Part model, mm, in its own coordinate system. A direction names the side the tool comes from. Round coordinates to 2 decimals unless told otherwise and drop trailing zeros. Loops run counter-clockwise (first coordinate to the right, second up) from the corner with the lowest first, then second, coordinate; pieces in that order, holes last.
1) Drop flat-ended pins along their axis: P1, Ø5.5, axis at x = -151.9, y = 9.59, coming from the -Z side; P2, Ø3, axis at y = -30.5, z = 19.5, coming from the +X side; P3, Ø2, axis at y = -24, z = 5.5, coming from the -X side; P4, Ø5.5, axis at x = -202.89, y = 41.4, coming from the +Z side. Give the stop position or say it passes through.
2) Band-saw the part on A-A, the plane z = 22. Write the cut outline in (x, y), then the cut area to 3 significant figures.
3) Mould opens along X. For faces 3 (the flat face through (-238.316, -10.619, 13.681)), 4 (the flat face through (-30, 12, 30)) say: +X half, -X half, draft (parallel to the pull), parting line (faces both ways), or undercut.
4) 3-axis set-ups, long thin cutter, end or side, ignore diameter. For faces 1 (the flat face through (18, 12, 0)), 2 (the flat face through (-193, 1, 27.75)): which of +Z, -Z, +X, -X, +Y, -Y reach the whole face in a straight line?
5) Probe line 1 (X direction, y = -2.5, z = 12); line 2 (Y direction, x = -189, z = 11); line 3 (X direction, y = -40, z = 24). List the from-to ranges inside material, lowest first.
6) Band-saw the part on B-B, the plane x = 116. Write the cut outline in (y, z).
7) Band-saw the part on C-C, the plane x = 17. Write the cut outline in (y, z), then the cut area to 3 significant figures.
from build123d import *

# Parameters (mm, degrees)
EXTRUDE_3_DEPTH     = 30
CUT_EXTRUDE_1_DEPTH = 27.75
SKETCH_5_R          = 1.75
CUT_EXTRUDE_2_DEPTH = 250.931131666


with BuildPart() as part:
    # 草图1 → 凸台-拉伸3 (new body)
    with BuildSketch(Plane.XY):
        with BuildLine():
            ThreePointArc((188.956439237, 0), (176.309013441, 23.14413618), (150, 25))
            Line((150, 25), (150, -25))
            ThreePointArc((150, -25), (176.309013441, -23.14413618), (188.956439237, 0))
        make_face()
        with BuildLine():
            Line((150, -25), (150, 25))
            ThreePointArc((150, 25), (133.956439237, 0), (150, -25))
        make_face()
        with BuildLine():
            ThreePointArc((188.956439237, 0), (176.309013441, 23.14413618), (150, 25))
            Line((150, 25), (150, -25))
            ThreePointArc((150, -25), (176.309013441, -23.14413618), (188.956439237, 0))
        make_face()
        with BuildLine():
            Line((150, -25), (150, 25))
            ThreePointArc((150, 25), (133.956439237, 0), (150, -25))
        make_face()
        with BuildLine():
            Line((150, 25), (-150, 25))
            ThreePointArc((-150, 25), (-145.004978875, 12.940952255), (-143.301270189, 0))
            ThreePointArc((-143.301270189, 0), (-145.004978875, -12.940952255), (-150, -25))
            ThreePointArc((-150, -25), (0, -7.455532034), (150, -25))
            ThreePointArc((150, -25), (133.956439237, 0), (150, 25))
        make_face()
        with BuildLine():
            ThreePointArc((-150, 25), (0, 41.260283441), (150, 25))
            Line((150, 25), (-150, 25))
        make_face()
        with BuildLine():
            ThreePointArc((-143.301270189, 0), (-145.004978875, 12.940952255), (-150, 25))
            Line((-150, 25), (-150, -25))
            ThreePointArc((-150, -25), (-145.004978875, -12.940952255), (-143.301270189, 0))
        make_face()
        with BuildLine():
            Line((-150, -25), (-150, 25))
            ThreePointArc((-150, 25), (-243.301270189, 0), (-150, -25))
        make_face()
        with BuildLine():
            ThreePointArc((-143.301270189, 0), (-145.004978875, 12.940952255), (-150, 25))
            Line((-150, 25), (-150, -25))
            ThreePointArc((-150, -25), (-145.004978875, -12.940952255), (-143.301270189, 0))
        make_face()
        with BuildLine():
            Line((-150, -25), (-150, 25))
            ThreePointArc((-150, 25), (-243.301270189, 0), (-150, -25))
        make_face()
    extrude(amount=EXTRUDE_3_DEPTH)

    # 草图3 → 切除-拉伸1 (cut)
    with BuildSketch(Plane(origin=(0, 0, 0), x_dir=(-1, 0, 0), z_dir=(0, 0, -1))):
        with BuildLine():
            ThreePointArc((241.460241998, 2.962420354), (203.950254971, 47.06019149), (151.10937756, 23.40740687))
            Line((151.10937756, 23.40740687), (145.115292459, -2.484763599))
            ThreePointArc((145.115292459, -2.484763599), (182.186192507, -46.952290127), (235.258997062, -23.8246019))
            Line((235.258997062, -23.8246019), (238.35961953, -10.431090773))
            Line((238.35961953, -10.431090773), (241.460241998, 2.962420354))
        make_face()
    extrude(amount=-CUT_EXTRUDE_1_DEPTH, mode=Mode.SUBTRACT)

    # 草图5 → 切除-拉伸2 (cut, through all)
    with BuildSketch(Plane(origin=(0, 0, 27.75), x_dir=(-1, 0, 0), z_dir=(0, 0, -1))):
        with Locations((151.896300525, 9.585326657)):
            Circle(SKETCH_5_R)
        with Locations((170.801384844, 36.055584303)):
            Circle(SKETCH_5_R)
        with Locations((202.886596846, 41.404969664)):
            Circle(SKETCH_5_R)
        with Locations((229.356854492, 22.499885346)):
            Circle(SKETCH_5_R)
        with Locations((234.706239853, -9.585326656)):
            Circle(SKETCH_5_R)
        with Locations((215.801155535, -36.055584303)):
            Circle(SKETCH_5_R)
        with Locations((183.715943533, -41.404969664)):
            Circle(SKETCH_5_R)
        with Locations((157.245685886, -22.499885346)):
            Circle(SKETCH_5_R)
    extrude(amount=-CUT_EXTRUDE_2_DEPTH, mode=Mode.SUBTRACT)


solid = part.part
Reported:
1. P1: stops at z = 27.75
1. P2: stops at x = -152.57
1. P3: stops at x = -237.7
1. P4: stops at z = 30
2. outline: (-150, -25) arc R650 cw to (150, -25) arc R27.5 ccw (long way) to (150, 25) arc R700 ccw to (-150, 25) arc R50 ccw (long way) to start; hole (-241.46, 2.96) - (-235.26, -23.82) arc R48.25 ccw to (-145.12, -2.48) - (-151.11, 23.41) arc R48.25 ccw to start
2. area: 16,900 mm2
3. face 3: undercut
3. face 4: draft
4. face 1: -Z, +X, -X, +Y, -Y
4. face 2: -Z
5. line 1: x = -243.24 to -240.2, -145.12 to 188.84
5. line 2: y = -49.81 to -48.06, 48.06 to 49.81
5. line 3: x = -223.3 to -220.28, -166.32 to -163.3
6. outline: (-17.89, 0) - (31.58, 0) - (31.58, 30) - (-17.89, 30) - close
7. outline: (-7.68, 0) - (41.05, 0) - (41.05, 30) - (-7.68, 30) - close
7. area: 1,460 mm2
